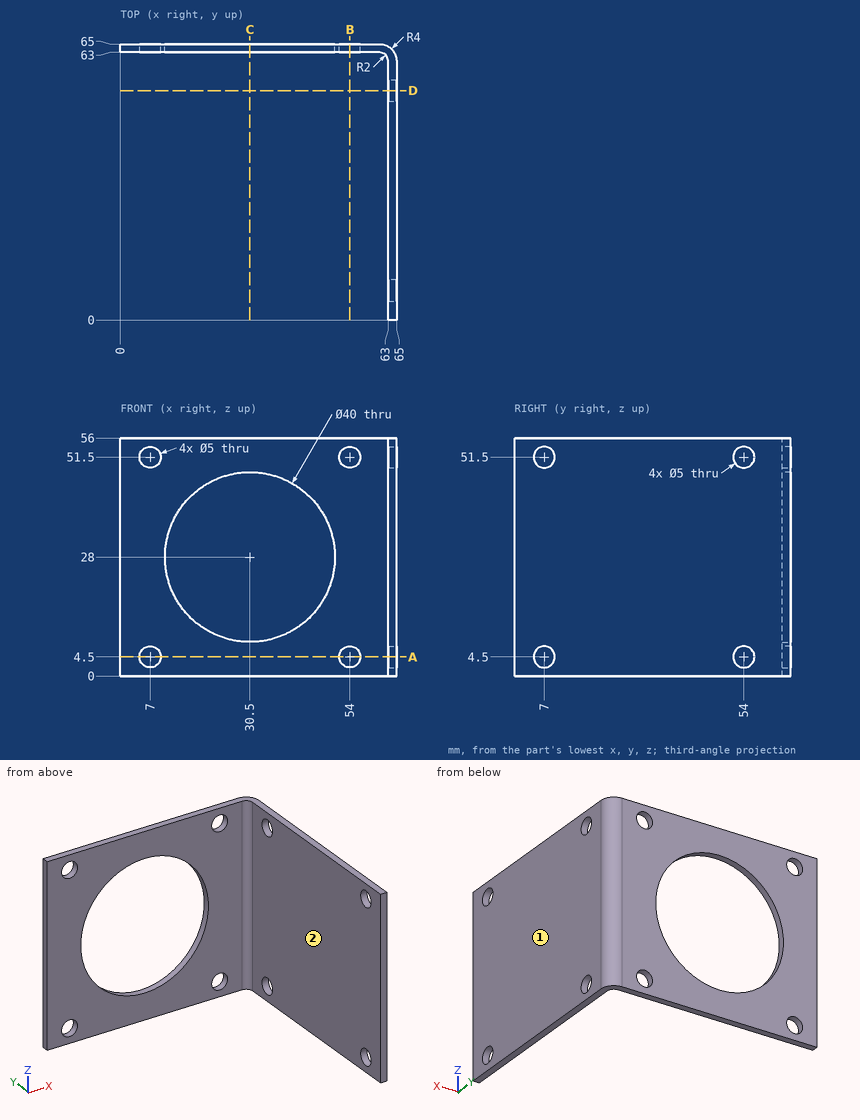
The figure shows three views and two pictorial views of one solid part (mm, origin at its lowest corner). Answer the questions. A direction names the side the tool comes from. Give positions to 0.01 mm unless a question says otherwise; leave off trailing zeros. Loops run counter-clockwise (first coordinate to the right, second up) from the corner with the lowest first, then second, coordinate; pieces in that order, holes last. Notation, with made-up numbers: (20.25, 22.25) -> (24.25, 22.25) arc R11 ccw to (24.25, 36.25) -> close; hole circle Ø3 at (-4.5, 36.25). An arc over 180 degrees is marked (long way). Use a Markdown table: item, result. Add a question column.
1. Section A-A on z = 4.5 is taken. Determine the outline of the cut face in (x, y).
2. For the marked faces 1 and 2, determine the directions among +Z, -Z, +X, -X, +Y, -Y from which every point of the face is accessible in a straight line to the end or side of a thin tool.
3. Find the intervals of material crossed by probe 1 along Z at (x, y) = (64.35, 7); probe 2 along X at (y, z) = (64, 51); probe 3 along X at (y, z) = (48, 24.5), in increasing order.
4. Flat-ended cylindrical pins translate along their axes: pin 1 Ø1 at (y, z) = (44, 46.5) entering from -X; pin 2 Ø4.5 at (x, z) = (54, 4.5) entering from +Y. Find the tip coordinate at first contact, or state that the pin passes through.
5. Section B-B on x = 54 is taken. Determine the outline of the cut face in (y, z), and give its area (3 significant figures).
6. Section C-C on x = 30.5 is taken. Determine the outline of the cut face in (y, z), and give its area (3 significant figures).
Results below:
| question | item | result |
|---|---|---|
| 1 | outline | (0, 63) -> (4.5, 63) -> (4.5, 65) -> (0, 65) -> close; (9.5, 63) -> (51.5, 63) -> (51.5, 65) -> (9.5, 65) -> close; (56.5, 63) -> (61, 63) arc R2 cw to (63, 61) -> (63, 56.5) -> (65, 56.5) -> (65, 61) arc R4 ccw to (61, 65) -> (56.5, 65) -> close; (63, 0) -> (65, 0) -> (65, 4.5) -> (63, 4.5) -> close; (63, 9.5) -> (65, 9.5) -> (65, 51.5) -> (63, 51.5) -> close |
| 2 | face 1 | +Z, -Z, +X, +Y, -Y |
| 2 | face 2 | +Z, -Z, -X, -Y |
| 3 | probe 1 | z = 0 to 2, 7 to 49, 54 to 56 |
| 3 | probe 2 | x = 0 to 4.55, 9.45 to 51.55, 56.45 to 63.65 |
| 3 | probe 3 | x = 63 to 65 |
| 4 | pin 1 | stops at x = 63 |
| 4 | pin 2 | passes through |
| 5 | outline | (63, 0) -> (65, 0) -> (65, 2) -> (63, 2) -> close; (63, 7) -> (65, 7) -> (65, 49) -> (63, 49) -> close; (63, 54) -> (65, 54) -> (65, 56) -> (63, 56) -> close |
| 5 | area | 92.0 mm^2 |
| 6 | outline | (63, 0) -> (65, 0) -> (65, 8) -> (63, 8) -> close; (63, 48) -> (65, 48) -> (65, 56) -> (63, 56) -> close |
| 6 | area | 32.0 mm^2 |
